```python
from build123d import *

# Parameters (mm, degrees)
CYLINDER008_R               = 6
CYLINDER008_DEPTH           = 20
CYLINDER008_PLACEMENT_ANGLE = 25
CYLINDER006_R               = 2
CYLINDER006_DEPTH           = 10
CYLINDER005_R               = 2
CYLINDER005_DEPTH           = 10
CYLINDER004_R               = 2
CYLINDER004_DEPTH           = 10
SKETCH_R                    = 10
EXTRUDE_DEPTH               = 2


with BuildPart() as cylinder008:
    # Cylinder008 → Cylinder008 (new body)
    with BuildSketch(Plane.XY):
        Circle(CYLINDER008_R)
    extrude(amount=CYLINDER008_DEPTH)


with BuildPart() as cylinder008_1:
    # Cylinder008 placement: moved
    add(cylinder008.part.moved(Location((-25, -20, -9))).rotate(Axis((-25, -20, -9), (0, -1, 0)), CYLINDER008_PLACEMENT_ANGLE))


with BuildPart() as cylinder006:
    # Cylinder006 → Cylinder006 (new body)
    with BuildSketch(Plane(origin=(-15, -36, -4), x_dir=(1, 0, 0), z_dir=(0, 0, 1))):
        Circle(CYLINDER006_R)
    extrude(amount=CYLINDER006_DEPTH)


with BuildPart() as cylinder005:
    # Cylinder005 → Cylinder005 (new body)
    with BuildSketch(Plane(origin=(10, -39, -4), x_dir=(1, 0, 0), z_dir=(0, 0, 1))):
        Circle(CYLINDER005_R)
    extrude(amount=CYLINDER005_DEPTH)


with BuildPart() as cylinder004:
    # Cylinder004 → Cylinder004 (new body)
    with BuildSketch(Plane(origin=(22, -22, -4), x_dir=(1, 0, 0), z_dir=(0, 0, 1))):
        Circle(CYLINDER004_R)
    extrude(amount=CYLINDER004_DEPTH)


with BuildPart() as cut007:
    # Sketch → Extrude (new body)
    with BuildSketch(Plane.XY):
        with BuildLine():
            Line((-55.05719, -35), (-27.221315, -35))
            ThreePointArc((-27.221315, -35), (10.719392, -46.318083), (34.94281, -15))
            Line((34.94281, 0), (34.94281, -15))
            Line((34.94281, 0), (-55.05719, 0))
            Line((-55.05719, -35), (-55.05719, 0))
        make_face()
        with Locations((0, -20)):
            Circle(SKETCH_R, mode=Mode.SUBTRACT)
    extrude(amount=EXTRUDE_DEPTH)

    # Cut004: cut Cylinder004
    add(cylinder004.part, mode=Mode.SUBTRACT)

    # Cut005: cut Cylinder005
    add(cylinder005.part, mode=Mode.SUBTRACT)

    # Cut006: cut Cylinder006
    add(cylinder006.part, mode=Mode.SUBTRACT)

    # Cut007: cut Cylinder008
    add(cylinder008_1.part, mode=Mode.SUBTRACT)


solid = cut007.part
```
Read the model definition and answer for the solid it produces. Units are mm, in the model's axes. A direction names the side the tool comes from. Give positions to 0.01 mm unless a question says otherwise; leave off trailing zeros. Write each loop counter-clockwise with the first axis right and the second up, starting at its lowest first coordinate (ties: lowest second). Pieces come first, ordered by that corner, then holes. Notation, with made-up numbers: M 63.25,66.25 L 116.25,66.25 A24 ccw 116.25,89.25 Z; hole C -17,6.5 d1. An arc over 180 degrees is marked long. Put each result on its own line as item: value. Start each with the question number.
1. Consider line 1 along X through (y, z) = (-22, 0.7); line 2 along X through (y, z) = (-15.5, 1.4); line 3 along Y through (x, z) = (0, 0.85). Determine where each line is inside the solid, lowest interval first.
2. This flat-tipped pin is pushed along its axis until it touches: pin 1 Ø12 at (x, y) = (0, -20) entering from -Z. Where does it stop, or does it pass through?
3. The part is cut by section D-D, the plane y = -16. Give the vertices of the cut face in (x, z).
4. For a pull along Y with two mould halves and no side action, classify faces 1 (the cylindrical face through (10.157, -46.494, 0.986)), 2 (the cylindrical face through (-15, -38, 1)), 3 (the flat face through (34.943, -7, 1)) as released by +Y, released by -Y, zero draft, split by the parting line, or undercut.
5. The part is cut by section C-C, the plane x = 22. Give the vertices of the cut face in (y, z).
6. Which of the six approach directions +Z, -Z, +X, -X, +Y, -Y give full straight-line access (tool end or side, diameter ignored) to faces 4 (the cylindrical face through (10, -41, 1)), 5 (the flat face through (-41, -35, 1))?
7. The part is cut by section B-B, the plane y = -39. Give the vertices of the cut face in (x, z), and give its area (3 significant figures).
8. The part is cut by section A-A, the plane y = -21. Give the vertices of the cut face in (x, z).
Final values:
1. line 1: x = -55.06 to -35.76, -23.28 to -9.8, 9.8 to 20, 24 to 33.82
1. line 2: x = -55.06 to -34.23, -25.47 to -8.93, 8.93 to 34.91
1. line 3: y = -48 to -30, -10 to 0
2. pin 1: passes through
3. outline: M -55.06,0 L -34.13,0 L -35.06,2 L -55.06,2 Z; M -25.19,2 L -24.26,0 L -9.17,0 L -9.17,2 Z; M 9.17,0 L 34.87,0 L 34.87,2 L 9.17,2 Z
4. face 1: released by -Y
4. face 2: undercut
4. face 3: zero draft
5. outline: M -40.22,0 L -24,0 L -24,2 L -40.22,2 Z; M -20,0 L 0,0 L 0,2 L -20,2 Z
6. face 4: +Z, -Z
6. face 5: +Z, -Z, -X, -Y
7. outline: M -23.43,0 L 8,0 L 8,2 L -23.43,2 Z; M 12,0 L 23.43,0 L 23.43,2 L 12,2 Z
7. area: 85.7 mm²
8. outline: M -55.06,0 L -35.72,0 L -36.66,2 L -55.06,2 Z; M -23.6,2 L -22.67,0 L -9.95,0 L -9.95,2 Z; M 9.95,0 L 20.27,0 L 20.27,2 L 9.95,2 Z; M 23.73,0 L 34.07,0 L 34.07,2 L 23.73,2 Z
